```python
from build123d import *

# Parameters (mm, degrees)
BOX003_W                 = 101.6
BOX003_H                 = 279.4
BOX003_DEPTH             = 12.7
BOX009_W                 = 12.7
BOX009_H                 = 44.1376
BOX009_DEPTH             = 139.7
BOX006_W                 = 12.7
BOX006_H                 = 44.1376
BOX006_DEPTH             = 139.7
BOX007_W                 = 12.7
BOX007_H                 = 44.1376
BOX007_DEPTH             = 139.7
SKETCH002_W              = 165.100117
SKETCH002_H              = 139.700117
SKETCH002_R              = 6.6548
SKETCH002_R_2            = 63.4873
PAD_DEPTH                = 12.7
CLONE001_PLACEMENT_ANGLE = 180
CLONE_PLACEMENT_ANGLE    = 180
BOX010_W                 = 165.1
BOX010_H                 = 12.7
BOX010_DEPTH             = 139.7
SKETCH004_R              = 63.4873
POCKET_DEPTH             = 12.7
BOX008_W                 = 12.7
BOX008_H                 = 44.1376
BOX008_DEPTH             = 139.7
BOX_W                    = 127
BOX_H                    = 114.3
BOX_DEPTH                = 139.7
BOX002_W                 = 12.7
BOX002_H                 = 279.4
BOX002_DEPTH             = 139.7


with BuildPart() as cube003:
    # Box003 → Box003 (new body)
    with BuildSketch(Plane(origin=(-224.636743, 494.971814, 58.555664), x_dir=(1, 0, 0), z_dir=(0, 0, 1))):
        with Locations((50.8, 139.7)):
            Rectangle(BOX003_W, BOX003_H)
    extrude(amount=BOX003_DEPTH)


with BuildPart() as cube009:
    # Box009 → Box009 (new body)
    with BuildSketch(Plane(origin=(-91.286743, 901.371814, -68.444336), x_dir=(1, 0, 0), z_dir=(0, 0, 1))):
        with Locations((6.35, 22.0688)):
            Rectangle(BOX009_W, BOX009_H)
    extrude(amount=BOX009_DEPTH)


with BuildPart() as cube006:
    # Box006 → Box006 (new body)
    with BuildSketch(Plane(origin=(-243.686743, 323.834214, -68.444336), x_dir=(1, 0, 0), z_dir=(0, 0, 1))):
        with Locations((6.35, 22.0688)):
            Rectangle(BOX006_W, BOX006_H)
    extrude(amount=BOX006_DEPTH)


with BuildPart() as cube007:
    # Box007 → Box007 (new body)
    with BuildSketch(Plane(origin=(-243.686743, 901.371814, -68.444336), x_dir=(1, 0, 0), z_dir=(0, 0, 1))):
        with Locations((6.35, 22.0688)):
            Rectangle(BOX007_W, BOX007_H)
    extrude(amount=BOX007_DEPTH)


with BuildPart() as pad:
    # Sketch002 → Pad (new body)
    with BuildSketch(Plane(origin=(0, 37.338, 0), x_dir=(-1, 0, 0), z_dir=(0, 1, 0))):
        with Locations((-69.215058, 89.86448)):
            Rectangle(SKETCH002_W, SKETCH002_H)
        with Locations((-121.408307, 142.057728)):
            Circle(SKETCH002_R, mode=Mode.SUBTRACT)
        with Locations((-17.02181, 142.057728)):
            Circle(SKETCH002_R, mode=Mode.SUBTRACT)
        with Locations((-17.02181, 37.671231)):
            Circle(SKETCH002_R, mode=Mode.SUBTRACT)
        with Locations((-121.408307, 37.671231)):
            Circle(SKETCH002_R, mode=Mode.SUBTRACT)
        with Locations((-69.215, 89.864421)):
            Circle(SKETCH002_R_2, mode=Mode.SUBTRACT)
    extrude(amount=PAD_DEPTH)


with BuildPart() as clone_of_pad001:
    # Clone001 base: copy of Pad
    add(pad.part)


with BuildPart() as clone_of_pad001_1:
    # Clone001 placement: moved
    add(clone_of_pad001.part.moved(Location((-91.921743, 995.547414, -88.458874))).rotate(Axis((-91.921743, 995.547414, -88.458874), (0, 0, 1)), CLONE001_PLACEMENT_ANGLE))


with BuildPart() as clone_of_pad:
    # Clone base: copy of Pad
    add(pad.part)


with BuildPart() as clone_of_pad_1:
    # Clone placement: moved
    add(clone_of_pad.part.moved(Location((-91.921626, 361.172214, -88.458874))).rotate(Axis((-91.921626, 361.172214, -88.458874), (0, 0, 1)), CLONE_PLACEMENT_ANGLE))


with BuildPart() as pocket:
    # Box010 → Box010 (new body)
    with BuildSketch(Plane(origin=(-102.435181, 88.203278, -436.376007), x_dir=(1, 0, 0), z_dir=(0, 0, 1))):
        with Locations((82.55, 6.35)):
            Rectangle(BOX010_W, BOX010_H)
    extrude(amount=BOX010_DEPTH)

    # Sketch004 → Pocket (cut)
    with BuildSketch(Plane(origin=(-102.435181, 88.203278, -436.376007), x_dir=(1, 0, 0), z_dir=(0, -1, 0))):
        with Locations((82.55, 69.85)):
            Circle(SKETCH004_R)
    extrude(amount=-POCKET_DEPTH, mode=Mode.SUBTRACT)


with BuildPart() as clone_of_pocket003005005:
    # Clone006 base: copy of Pocket
    add(pocket.part)


with BuildPart() as clone_of_pocket003005005_1:
    # Clone006 placement: moved
    add(clone_of_pocket003005005.part.moved(Location((-141.251562, 800.468536, 367.931671))))


with BuildPart() as clone_of_pocket:
    # Clone005 base: copy of Pocket
    add(pocket.part)


with BuildPart() as clone_of_pocket_1:
    # Clone005 placement: moved
    add(clone_of_pocket.part.moved(Location((-141.251562, 279.768536, 367.931671))))


with BuildPart() as cube008:
    # Box008 → Box008 (new body)
    with BuildSketch(Plane(origin=(-91.286743, 323.834214, -68.444336), x_dir=(1, 0, 0), z_dir=(0, 0, 1))):
        with Locations((6.35, 22.0688)):
            Rectangle(BOX008_W, BOX008_H)
    extrude(amount=BOX008_DEPTH)


with BuildPart() as cube:
    # Box → Box (new body)
    with BuildSketch(Plane(origin=(-224.636743, 380.671814, -68.444336), x_dir=(1, 0, 0), z_dir=(0, 0, 1))):
        with Locations((63.5, 57.15)):
            Rectangle(BOX_W, BOX_H)
    extrude(amount=BOX_DEPTH)


with BuildPart() as clone_of_cube:
    # Clone008 base: copy of Cube
    add(cube.part)


with BuildPart() as clone_of_cube_1:
    # Clone008 placement: moved
    add(clone_of_cube.part.moved(Location((0, 393.7, 0))))


with BuildPart() as fusion:
    # Box002 → Box002 (new body)
    with BuildSketch(Plane(origin=(-123.036743, 494.971814, -68.444336), x_dir=(1, 0, 0), z_dir=(0, 0, 1))):
        with Locations((6.35, 139.7)):
            Rectangle(BOX002_W, BOX002_H)
    extrude(amount=BOX002_DEPTH)

    # Fusion: union Cube003, Cube009, Cube006, Cube007, Clone of Pad001, Clone of Pad, Clone of Pocket003005005, Clone of Pocket, Cube008, Clone of Cube, Cube
    add(cube003.part)
    add(cube009.part)
    add(cube006.part)
    add(cube007.part)
    add(clone_of_pad001_1.part)
    add(clone_of_pad_1.part)
    add(clone_of_pocket003005005_1.part)
    add(clone_of_pocket_1.part)
    add(cube008.part)
    add(clone_of_cube_1.part)
    add(cube.part)


solid = fusion.part
```
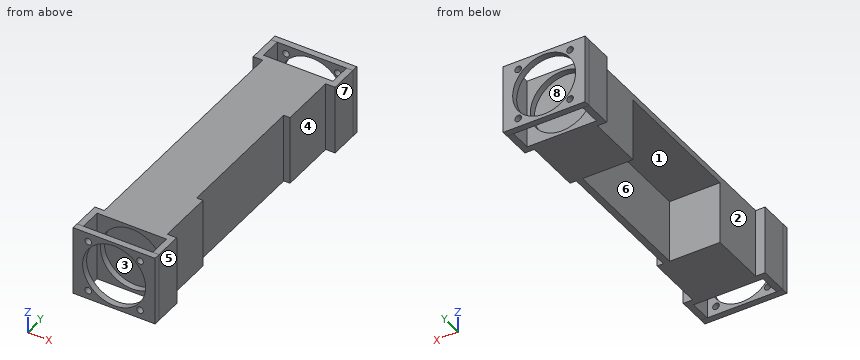
Geometry: final body of the model. Coordinates: model frame, mm. Face numbers are marked on the shaded views. A direction names the side the tool comes from. Round coordinates to 2 decimals unless told otherwise and drop trailing zeros. Order: outer loops, then holes, each group sorted by start corner. A loop starts at its lowest first (then second) coordinate and runs counter-clockwise, first axis right, second up. Notation, with made-up numbers: M -26,67 L 29,67 A19 cw 29,77 Z; hole C -27,27.25 d9. An arc over 180 degrees is marked long. Use one line per item in the form item = value. Start each with the question number.
Q1. Access query for the marked faces 1, 2, 3, 4 and 5. Directions: +Z, -Z, +X, -X, +Y, -Y. A direction counts if a zero-diameter tool reaches every point of the face in a straight line with its end or side. Return the directions, or none.
Q2. Material intervals for line 1 (Y direction, x = -206.5, z = 56.5); line 2 (Y direction, x = -93.5, z = 40); line 3 (X direction, y = 339, z = 39.5), sorted ascending. Write a range as [from, to].
Q3. Pin query (flat end, axial travel): pin 1 Ø10.5 at (x, z) = (-108.94, -50.79) entering from -Y; pin 2 Ø4 at (x, z) = (-165, 38.5) entering from +Y; pin 3 Ø1.5 at (y, z) = (439, -14) entering from -X; pin 4 Ø3 at (x, y) = (-107.5, 639.5) entering from -Z. Return the tip coordinate at first contact, or that it passes through.
Q4. Cut plane B-B (x = -157.5). Count the separate pieces of the cut face and the enclosed holes in it, and give its area (3 significant figures).
Q5. Cut plane A-A (y = 360). Return loops of the section in (x, z).
Q6. Mould query, pull axis Y, two halves, no side actions, for the marked faces 6, 7 and 8. Classes: +Y half, -Y half, draft (parallel to the pull), parting line (faces both ways), or undercut.
Q7. Cut plane C-C (y = 518). Return loops of the section in (x, z).
Geometry results:
q1.face_1 = -Z, -X
q1.face_2 = +Z, -Z, -X
q1.face_3 = -Y
q1.face_4 = +Z, -Z, +X
q1.face_5 = +Z, -Z, +X, +Y, -Y
q2.line_1 = [311.13, 323.83], [367.97, 494.97], [774.37, 901.37], [945.51, 958.21]
q2.line_2 = [311.13, 323.83], [367.97, 380.67], [888.67, 901.37], [945.51, 958.21]
q2.line_3 = [-243.69, -230.99], [-91.29, -78.59]
q3.pin_1 = 367.97
q3.pin_2 = 888.67
q3.pin_3 = -224.64
q3.pin_4 = through
q4.separate_pieces = 5
q4.enclosed_holes = 0
q4.area = 36,100 mm^2
q5.outline = M -243.69,-68.44 L -230.99,-68.44 L -230.99,71.26 L -243.69,71.26 Z; M -91.29,-68.44 L -78.59,-68.44 L -78.59,71.26 L -91.29,71.26 Z
q6.face_6 = undercut
q6.face_7 = draft
q6.face_8 = +Y half
q7.outline = M -224.64,58.56 L -123.04,58.56 L -123.04,-68.44 L -110.34,-68.44 L -110.34,71.26 L -224.64,71.26 Z
